The model under review builds one solid part; all positions refer to its coordinate system, in mm. Face numbers are marked on the shaded views. A direction names the side the tool comes from. Give positions to 0.01 mm unless a question says otherwise; leave off trailing zeros. Loops run counter-clockwise (first coordinate to the right, second up) from the corner with the lowest first, then second, coordinate; pieces in that order, holes last. Notation, with made-up numbers: (-32, 50) - (-28, 50) arc R29 ccw to (-28, 87) - close; hole circle Ø3 at (28.25, 73.5). An arc over 180 degrees is marked (long way). Answer as a JSON object with one key per item and string values.
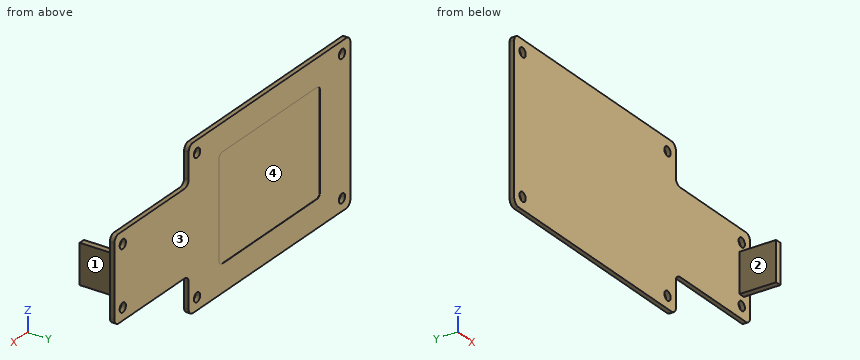
from build123d import *

# Parameters (mm, degrees)
BOSS_EXTRUDE1_DEPTH     = 0.75
FILLET1_R               = 2
SKETCH2_R               = 1.5
CUT_EXTRUDE1_DEPTH      = 1.5
CUT_EXTRUDE2_DEPTH      = 0.1
CUT_EXTRUDE2_DEPTH_BACK = 0.1
SKETCH5_W               = 2
SKETCH5_H               = 13
BOSS_EXTRUDE2_DEPTH     = 12


with BuildPart() as part:
    # Sketch1 → Boss-Extrude1 (new, symmetric)
    with BuildSketch(Plane(origin=(0, 0, 0), x_dir=(1, 0, 0), z_dir=(0, 1, 0))):
        Polygon((-38.65, 26.15), (38.65, 26.15), (38.65, 13.75), (74.15, 13.75), (74.15, -13.75), (38.65, -13.75), (38.65, -26.15), (-38.65, -26.15), align=None)
    extrude(amount=BOSS_EXTRUDE1_DEPTH, both=True)

    # Fillet1
    fillet1_edges = [part.edges().sort_by_distance(p)[0] for p in [
        (38.65, 0, -13.75),
        (74.15, 0, -13.75),
        (74.15, 0, 13.75),
        (38.65, 0, 13.75),
        (38.65, 0, 26.15),
        (-38.65, 0, 26.15),
        (-38.65, 0, -26.15),
        (38.65, 0, -26.15),
    ]]
    fillet(fillet1_edges, radius=FILLET1_R)

    # Sketch2 → Cut-Extrude1 (cut)
    with BuildSketch(Plane(origin=(0, 0.75, 0), x_dir=(1, 0, 0), z_dir=(0, 1, 0))):
        with Locations(Location((-34.65, 22.15, 0), (0, 0, 270))):
            Circle(SKETCH2_R)
        with Locations(Location((34.65, 22.15, 0), (0, 0, 270))):
            Circle(SKETCH2_R)
        with Locations(Location((34.65, -22.15, 0), (0, 0, 270))):
            Circle(SKETCH2_R)
        with Locations(Location((-34.65, -22.15, 0), (0, 0, 270))):
            Circle(SKETCH2_R)
        with Locations(Location((70.15, 9.75, 0), (0, 0, 270))):
            Circle(SKETCH2_R)
        with Locations(Location((70.15, -9.75, 0), (0, 0, 270))):
            Circle(SKETCH2_R)
    extrude(amount=-CUT_EXTRUDE1_DEPTH, mode=Mode.SUBTRACT)

    # Sketch4 → Cut-Extrude2 (cut, two sides: drawn at the far end of the back side and taken through both)
    with BuildSketch(Plane(origin=(0, 0.75, 0), x_dir=(1, 0, 0), z_dir=(0, 1, 0)).offset(-CUT_EXTRUDE2_DEPTH_BACK)):
        with BuildLine():
            Line((-22.65, 17.15), (22.65, 17.15))
            ThreePointArc((22.65, 17.15), (23.710660172, 16.710660172), (24.15, 15.65))
            Line((24.15, 15.65), (24.15, -15.65))
            ThreePointArc((24.15, -15.65), (23.710660172, -16.710660172), (22.65, -17.15))
            Line((22.65, -17.15), (-22.65, -17.15))
            ThreePointArc((-22.65, -17.15), (-23.710660172, -16.710660172), (-24.15, -15.65))
            Line((-24.15, -15.65), (-24.15, 15.65))
            ThreePointArc((-24.15, 15.65), (-23.710660172, 16.710660172), (-22.65, 17.15))
        make_face()
    extrude(amount=CUT_EXTRUDE2_DEPTH + CUT_EXTRUDE2_DEPTH_BACK, mode=Mode.SUBTRACT)

    # Sketch5 → Boss-Extrude2 (add)
    with BuildSketch(Plane.XZ.offset(0.75)):
        with Locations((70.15, 0)):
            Rectangle(SKETCH5_W, SKETCH5_H)
    extrude(amount=BOSS_EXTRUDE2_DEPTH)


solid = part.part
Q1. The part is to be moulded in two halves that separate along Z. For the marked faces 3 and 4, say which applies: +Z half, -Z half, draft (parallel to the pull), parting line (faces both ways), or undercut.
Results:
{"face 3": "draft", "face 4": "undercut"}
Q2. Consider section D-D, the plane x = -13.5. State the section outline as (y, z) points, plus the area to 3 significant figures.
Results:
{"outline": "(-0.75, -26.15) - (0.75, -26.15) - (0.75, -17.15) - (0.65, -17.15) - (0.65, 17.15) - (0.75, 17.15) - (0.75, 26.15) - (-0.75, 26.15) - close", "area": "75.0 mm^2"}
Q3. Consider section A-A, the plane x = -34.65. State the section outline as (y, z) points.
Results:
{"outline": "(-0.75, -26.15) - (0.75, -26.15) - (0.75, -23.65) - (-0.75, -23.65) - close; (-0.75, -20.65) - (0.75, -20.65) - (0.75, 20.65) - (-0.75, 20.65) - close; (-0.75, 23.65) - (0.75, 23.65) - (0.75, 26.15) - (-0.75, 26.15) - close"}
Q4. Clearance check with flat-ended pins moving along their axes: pin 1 Ø1.6 at (x, y) = (60, 0) entering from -Z; pin 2 Ø3 at (x, z) = (10, 15) entering from +Y; pin 3 Ø1.5 at (x, y) = (60.5, -1) entering from +Z. State where each tip first meets the part, or that it passes through.
Results:
{"pin 1": "stops at z = -13.75", "pin 2": "stops at y = 0.65", "pin 3": "stops at z = 13.75"}
Q5. For the marked faces 1 and 2, list the 3-axis set-ups (+Z, -Z, +X, -X, +Y, -Y) from which the entire face can be reached by the end or side of a thin tool; tool diameter is ignored.
Results:
{"face 1": "+Z, -Z, +X, -Y", "face 2": "+Z, -Z, -X, -Y"}
Q6. To check wall thickness, follow probe 1 along X at (y, z) = (0.1, -22.15); probe 2 along Z at (x, y) = (70.15, -0.2); probe 3 along X at (y, z) = (-0.2, 9.75). State the ranges of each line that lie inside material, in increasing order. Write a range as [from, to].
Results:
{"probe 1": "x = [-38.65, -36.15], [-33.15, 33.15], [36.15, 38.65]", "probe 2": "z = [-13.75, -11.25], [-8.25, 8.25], [11.25, 13.75]", "probe 3": "x = [-38.65, 68.65], [71.65, 74.15]"}
Q7. Consider section C-C, the plane z = -22.15. State the section outline as (x, y) points.
Results:
{"outline": "(-38.65, -0.75) - (-36.15, -0.75) - (-36.15, 0.75) - (-38.65, 0.75) - close; (-33.15, -0.75) - (33.15, -0.75) - (33.15, 0.75) - (-33.15, 0.75) - close; (36.15, -0.75) - (38.65, -0.75) - (38.65, 0.75) - (36.15, 0.75) - close"}
Q8. Consider section B-B, the plane z = 9.75. State the section outline as (x, y) points, plus the area to 3 significant figures.
Results:
{"outline": "(-38.65, -0.75) - (68.65, -0.75) - (68.65, 0.75) - (24.15, 0.75) - (24.15, 0.65) - (-24.15, 0.65) - (-24.15, 0.75) - (-38.65, 0.75) - close; (71.65, -0.75) - (74.15, -0.75) - (74.15, 0.75) - (71.65, 0.75) - close", "area": "160 mm^2"}
